```python
from build123d import *

# Parameters (mm, degrees)
F0_W     = 38.1
F0_H     = 76.2
F1_DEPTH = 1028.7
F2_T     = -2.778125
F3_R     = 3.175
F4_DEPTH = 38.101
F5_R     = 3.175
F6_DEPTH = 2057.401
F7_R     = 2.579688
F8_DEPTH = 76.201


with BuildPart() as f1:
    # F0 (on Top) → F1 (new body, symmetric)
    with BuildSketch(Plane.XY):
        with Locations((19.05, 38.1)):
            Rectangle(F0_W, F0_H)
    extrude(amount=F1_DEPTH, both=True)

    # F2
    f2_openings = [f1.faces().sort_by_distance(p)[0] for p in [
        (38.1, 38.1, 0),
    ]]
    offset(amount=F2_T, openings=f2_openings)

    # F3 (on face) → F4 (cut, through all)
    with BuildSketch(Plane(origin=(0, 0, 0), x_dir=(0, -1, 0), z_dir=(-1, 0, 0))):
        with Locations((-63.5, -946.15)):
            Circle(F3_R)
        with Locations((-12.7, -946.15)):
            Circle(F3_R)
        with Locations((-63.5, -412.75)):
            Circle(F3_R)
        with Locations((-12.7, -412.75)):
            Circle(F3_R)
        with Locations((-63.5, 120.65)):
            Circle(F3_R)
        with Locations((-12.7, 120.65)):
            Circle(F3_R)
        with Locations((-63.5, 654.05)):
            Circle(F3_R)
        with Locations((-12.7, 654.05)):
            Circle(F3_R)
    extrude(amount=-F4_DEPTH, mode=Mode.SUBTRACT)

    # F5 (on face) → F6 (cut, through all)
    with BuildSketch(Plane(origin=(0, 0, -1028.7), x_dir=(1, 0, 0), z_dir=(0, 0, -1))):
        with Locations((19.05, -12.7)):
            Circle(F5_R)
        with Locations((19.05, -63.5)):
            Circle(F5_R)
    extrude(amount=-F6_DEPTH, mode=Mode.SUBTRACT)

    # F7 (on face) → F8 (cut, through all)
    with BuildSketch(Plane(origin=(0, 76.2, 0), x_dir=(-1, 0, 0), z_dir=(0, 1, 0))):
        with Locations((-19.05, 561.975)):
            Circle(F7_R)
        with Locations((-19.05, 511.175)):
            Circle(F7_R)
        with Locations((-19.05, 133.35)):
            Circle(F7_R)
        with Locations((-19.05, -22.225)):
            Circle(F7_R)
        with Locations((-19.05, 28.575)):
            Circle(F7_R)
        with Locations((-19.05, -400.05)):
            Circle(F7_R)
        with Locations((-19.05, -555.625)):
            Circle(F7_R)
        with Locations((-19.05, -504.825)):
            Circle(F7_R)
        with Locations((-19.05, -933.45)):
            Circle(F7_R)
        with Locations((-19.05, 666.75)):
            Circle(F7_R)
        with Locations((-19.05, 1009.65)):
            Circle(F7_R)
    extrude(amount=-F8_DEPTH, mode=Mode.SUBTRACT)


solid = f1.part
```
Check sheet for the modelled part. Datum: model origin and axes. Units: mm. A direction names the side the tool comes from. Give positions to 0.01 mm unless a question says otherwise; leave off trailing zeros. Write each loop counter-clockwise with the first axis right and the second up, starting at its lowest first coordinate (ties: lowest second). Pieces come first, ordered by that corner, then holes.
Item 1: Access from +Z, -Z, +X, -X, +Y, -Y to the whole of each face (thin tool, end or side, straight path). Record for faces 4 (the face through (19, 39, 1028.7)), 5 (the face through (20, 39, 1025.922)).
Item 2: Scan lines: L1, parallel to Y at x = 19.05, z = 1028.05 (3 decimals); L2, parallel to Z at x = 4.5, y = 44; L3, parallel to X at y = 74, z = 133. Record each from-to range of solid material in increasing order.
Item 3: Gauge pin test, flat ends, axial feed: pin 1 (6 mm diameter, centred on y = 49, z = -690.5, fed in from -X); pin 2 (8 mm diameter, centred on y = 30.5, z = -277.5, fed in from +X). Record the tip position at first contact, or that the pin passes through.
Item 4: Draft check along Z on faces 1 (the face through (38.1, 1, 5)), 2 (the face through (20, 39, -1025.922)), 3 (the face through (19, 39, -1028.7)). Enter one of: released by +Z, released by -Z, zero draft, split by the parting line, or undercut.
Item 5: Cross-section at A-A (z = 797). Enter the section's corners in (x, y).
Item 6: Cross-section at B-B (y = 36). Enter the section's corners in (x, z).
Report:
1. face 4: +Z, +X, -X, +Y, -Y
1. face 5: +X
2. L1: y = 0 to 9.525, 15.875 to 60.325, 66.675 to 76.2
2. L2: z = -1028.7 to -1025.92, 1025.92 to 1028.7
2. L3: x = 0 to 16.49, 21.61 to 38.1
3. pin 1: stops at x = 0
3. pin 2: stops at x = 2.78
4. face 1: zero draft
4. face 2: undercut
4. face 3: released by -Z
5. outline: (0, 0) - (38.1, 0) - (38.1, 2.78) - (2.78, 2.78) - (2.78, 73.42) - (38.1, 73.42) - (38.1, 76.2) - (0, 76.2) - close
6. outline: (0, -1028.7) - (38.1, -1028.7) - (38.1, -1025.92) - (2.78, -1025.92) - (2.78, 1025.92) - (38.1, 1025.92) - (38.1, 1028.7) - (0, 1028.7) - close
